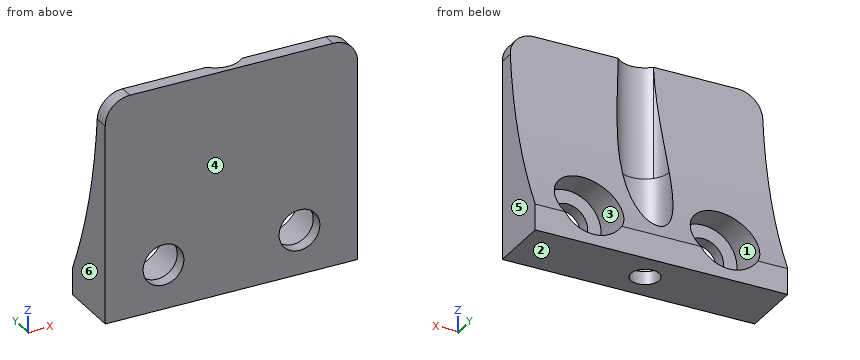
from build123d import *

# Parameters (mm, degrees)
SKETCH1_W                       = 20.45
SKETCH1_H                       = 18.1
BOSS_EXTRUDE2_DEPTH             = 1
BOSS_EXTRUDE3_REACH             = 15.691
BOSS_EXTRUDE3_DIRECTION_2_REACH = 15.691
SKETCH4_R                       = 1.65
CUT_EXTRUDE1_DEPTH              = 5
BOSS_EXTRUDE5_START             = -10.225
BOSS_EXTRUDE5_DEPTH             = 20.45
SKETCH6_R                       = 2.75
CUT_EXTRUDE2_DEPTH              = 4
SKETCH7_R                       = 1.15
CUT_EXTRUDE3_DEPTH              = 9.05
SKETCH8_R                       = 2
CUT_EXTRUDE4_DEPTH              = 8
CUT_EXTRUDE4_DIRECTION_2_REACH  = 16.541
FILLET1_R                       = 2


with BuildPart() as part:
    # Sketch1 → Boss-Extrude2 (new body)
    with BuildSketch(Plane(origin=(0, 0, 0), x_dir=(1, 0, 0), z_dir=(0, 1, 0))):
        Rectangle(SKETCH1_W, SKETCH1_H)
    extrude(amount=BOSS_EXTRUDE2_DEPTH)

    # Boss-Extrude3: up to this face of the body (flat: up to its plane)
    boss_extrude3_end = Plane(part.part.faces().sort_by_distance((10.225, 0.5, 0))[0])
    # Sketch3 → Boss-Extrude3 (add, up to the picked face)
    with BuildSketch(Plane(origin=(0, 0, 0), x_dir=(0, 0, -1), z_dir=(1, 0, 0)), mode=Mode.PRIVATE) as boss_extrude3_sk1:
        Polygon((9.05, 1), (9.05, 5), (7.05, 5), (3.05, 1), align=None)
    boss_extrude3_tool1 = split(extrude(boss_extrude3_sk1.sketch, amount=BOSS_EXTRUDE3_REACH, mode=Mode.PRIVATE), bisect_by=boss_extrude3_end, keep=Keep.BOTH, mode=Mode.PRIVATE)
    add(boss_extrude3_tool1.solids().sort_by(Axis((0, 2.666667, -6.883333), (1, 0, 0)))[0])

    # Boss-Extrude3 direction 2: up to this face of the body (flat: up to its plane)
    boss_extrude3_direction_2_end = Plane(part.part.faces().sort_by_distance((-10.225, 0.5, 0))[0])
    # Sketch3 → Boss-Extrude3 direction 2 (add, up to the picked face)
    with BuildSketch(Plane(origin=(0, 0, 0), x_dir=(0, 0, -1), z_dir=(1, 0, 0)), mode=Mode.PRIVATE) as boss_extrude3_direction_2_sk1:
        Polygon((9.05, 1), (9.05, 5), (7.05, 5), (3.05, 1), align=None)
    boss_extrude3_direction_2_tool1 = split(extrude(boss_extrude3_direction_2_sk1.sketch, amount=-BOSS_EXTRUDE3_DIRECTION_2_REACH, mode=Mode.PRIVATE), bisect_by=boss_extrude3_direction_2_end, keep=Keep.BOTH, mode=Mode.PRIVATE)
    add(boss_extrude3_direction_2_tool1.solids().sort_by(Axis((0, 2.666667, -6.883333), (-1, 0, 0)))[0])

    # Sketch4 → Cut-Extrude1 (cut)
    with BuildSketch(Plane(origin=(0, 5, 0), x_dir=(1, 0, 0), z_dir=(0, 1, 0))):
        with Locations(Location((-5.505, 5.45, 0), (0, 0, 104.141110234))):
            Circle(SKETCH4_R)
        with Locations(Location((5.505, 5.45, 0), (0, 0, 75.858889766))):
            Circle(SKETCH4_R)
    extrude(amount=-CUT_EXTRUDE1_DEPTH, mode=Mode.SUBTRACT)

    # Sketch10 → Boss-Extrude5 (add)
    with BuildSketch(Plane(origin=(0, 0, 0), x_dir=(0, 0, -1), z_dir=(1, 0, 0)).offset(BOSS_EXTRUDE5_START)):
        with BuildLine():
            Line((3.05, 1), (7.05, 5))
            Line((7.05, 5), (6.95, 5))
            ThreePointArc((6.95, 5), (-0.847118083, 2.217663929), (-9.05, 1.1))
            Line((-9.05, 1.1), (-9.05, 1))
            Line((-9.05, 1), (3.05, 1))
        make_face()
    extrude(amount=BOSS_EXTRUDE5_DEPTH)

    # Sketch6 → Cut-Extrude2 (cut)
    with BuildSketch(Plane(origin=(0, 5, 0), x_dir=(1, 0, 0), z_dir=(0, 1, 0))):
        with Locations(Location((-5.505, 5.45, 0), (0, 0, 270))):
            Circle(SKETCH6_R)
        with Locations(Location((5.505, 5.45, 0), (0, 0, 270))):
            Circle(SKETCH6_R)
    extrude(amount=-CUT_EXTRUDE2_DEPTH, mode=Mode.SUBTRACT)

    # Sketch7 → Cut-Extrude3 (cut)
    with BuildSketch(Plane.XY):
        with Locations((0, 2.5)):
            Circle(SKETCH7_R)
    extrude(amount=-CUT_EXTRUDE3_DEPTH, mode=Mode.SUBTRACT)

    # Sketch8 → Cut-Extrude4 (cut)
    with BuildSketch(Plane.XY):
        with Locations(Location((0, 2.5, 0), (0, 0, 224.427004001))):
            Circle(SKETCH8_R)
    extrude(amount=-CUT_EXTRUDE4_DEPTH, mode=Mode.SUBTRACT)

    # Cut-Extrude4 direction 2: up to this face of the body (flat: up to its plane)
    cut_extrude4_direction_2_end = Plane(part.part.faces().sort_by_distance((0, 0.55, 9.05))[0])
    # Sketch8 → Cut-Extrude4 direction 2 (cut, up to the picked face)
    with BuildSketch(Plane.XY, mode=Mode.PRIVATE) as cut_extrude4_direction_2_sk1:
        with Locations(Location((0, 2.5, 0), (0, 0, 224.427004001))):
            Circle(SKETCH8_R)
    cut_extrude4_direction_2_tool1 = split(extrude(cut_extrude4_direction_2_sk1.sketch, amount=CUT_EXTRUDE4_DIRECTION_2_REACH, mode=Mode.PRIVATE), bisect_by=cut_extrude4_direction_2_end, keep=Keep.BOTH, mode=Mode.PRIVATE)
    add(cut_extrude4_direction_2_tool1.solids().sort_by(Axis((0, 2.5, 0), (0, 0, 1)))[0], mode=Mode.SUBTRACT)

    # Fillet1
    fillet1_edges = [part.edges().sort_by_distance(p)[0] for p in [
        (10.225, 0.55, 9.05),
        (-10.225, 0.55, 9.05),
    ]]
    fillet(fillet1_edges, radius=FILLET1_R)


solid = part.part
Input: part model. Units: mm. Frame: model coordinates. Face numbers are marked on the shaded views. A direction names the side the tool comes from. Coordinates: 2 decimals unless noted, no trailing zeros. Loops run counter-clockwise (first coordinate to the right, second up) from the corner with the lowest first, then second, coordinate; pieces in that order, holes last.
Q1. Cut plane B-B (z = -5.45). Output: boundary loops of the cut face in (x, y) (3 decimals).
Q2. Cut plane C-C (y = 3.9). Output: boundary loops of the cut face in (x, z) (3 decimals), then the cut area to 3 significant figures.
Q3. Cut plane A-A (x = 0). Output: boundary loops of the cut face in (y, z), then the cut area to 3 significant figures.
Q4. Set-up query: the marked faces 1 and 2. Return all of +Z, -Z, +X, -X, +Y, -Y with unobstructed straight access to the full face (end or side cutting, diameter ignored); none if empty.
Q5. Contact query for flat-ended pins moving along their axis: pin 1 (1 mm diameter, centred on x = -0.5, z = -3, fed in from +Y); pin 2 (1 mm diameter, centred on x = -7, z = 0, fed in from +Y); pin 3 (3 mm diameter, centred on x = 0, y = 2.5, fed in from +Z); pin 4 (2 mm diameter, centred on x = -5.505, z = -5.45, fed in from -Y). Output: stop coordinate, or through.
Q6. Draft query along X for the marked faces 3, 4, 5 and 6. Return one class per face: +X half, -X half, draft (parallel to the pull), parting line (faces both ways), or undercut.
Q7. Cut plane D-D (z = -3). Output: boundary loops of the cut face in (x, y) (3 decimals), then the cut area to 3 significant figures.
Q8. Material intervals for line 1 (X direction, y = 0.2, z = -5.45) (3 decimals); line 2 (X direction, y = 0.9, z = -5.25) (3 decimals); line 3 (X direction, y = 2.65, z = -4) (3 decimals), sorted ascending.
Working result:
1. outline: (-10.225, 0) - (-7.155, 0) - (-7.155, 1) - (-8.255, 1) - (-8.255, 4.32) - (-10.225, 4.32) - close; (-3.855, 0) - (3.855, 0) - (3.855, 1) - (2.755, 1) - (2.755, 4.32) - (0.83, 4.32) arc R2 cw (long way) to (-0.83, 4.32) - (-2.755, 4.32) - (-2.755, 1) - (-3.855, 1) - close; (7.155, 0) - (10.225, 0) - (10.225, 4.32) - (8.255, 4.32) - (8.255, 1) - (7.155, 1) - close
2. outline: (-10.225, -9.05) - (10.225, -9.05) - (10.225, -4.434) - (8.06, -4.434) arc R2.75 cw (long way) to (2.95, -4.434) - (1.428, -4.434) - (1.428, -8) - (-1.428, -8) - (-1.428, -4.434) - (-2.95, -4.434) arc R2.75 cw (long way) to (-8.06, -4.434) - (-10.225, -4.434) - close
2. area: 49.5 mm2
3. outline: (0, -9.05) - (1.35, -9.05) - (1.35, -8) - (0.5, -8) - (0.5, 9.05) - (0, 9.05) - close; (3.65, -9.05) - (5, -9.05) - (5, -6.95) arc R40 cw to (4.5, -5.86) - (4.5, -8) - (3.65, -8) - close
3. area: 12.2 mm2
4. face 1: +Y
4. face 2: -Z, +X, -X, +Y, -Y
5. pin 1: stops at y = 0.77
5. pin 2: stops at y = 2.57
5. pin 3: stops at z = -8
5. pin 4: passes through
6. face 3: undercut
6. face 4: draft
6. face 5: +X half
6. face 6: -X half
7. outline: (-10.225, 0) - (10.225, 0) - (10.225, 3.363) - (6.754, 3.363) - (6.754, 1) - (4.256, 1) - (4.256, 3.363) - (1.804, 3.363) arc R2 cw (long way) to (-1.804, 3.363) - (-4.256, 3.363) - (-4.256, 1) - (-6.754, 1) - (-6.754, 3.363) - (-10.225, 3.363) - close
7. area: 47.3 mm2
8. line 1: x = -10.225 to -7.155, -3.855 to 3.855, 7.155 to 10.225
8. line 2: x = -10.225 to -7.143, -3.867 to -1.2, 1.2 to 3.867, 7.143 to 10.225
8. line 3: x = -10.225 to -7.842, -3.168 to -1.994, 1.994 to 3.168, 7.842 to 10.225
